The drawing under review shows one solid part. Ordinate dimensions are in mm from its lowest x, y, z. Round coordinates to 2 decimals unless told otherwise and drop trailing zeros. Order: outer loops, then holes, each group sorted by start corner. A loop starts at its lowest first (then second) coordinate and runs counter-clockwise, first axis right, second up. Notation, with made-up numbers: M 3,80 L 17,80 A24 ccw 17,114 Z; hole C 61,1.5 d8. An arc over 180 degrees is marked long. Answer in a Markdown table with one row per item. Add a question column.
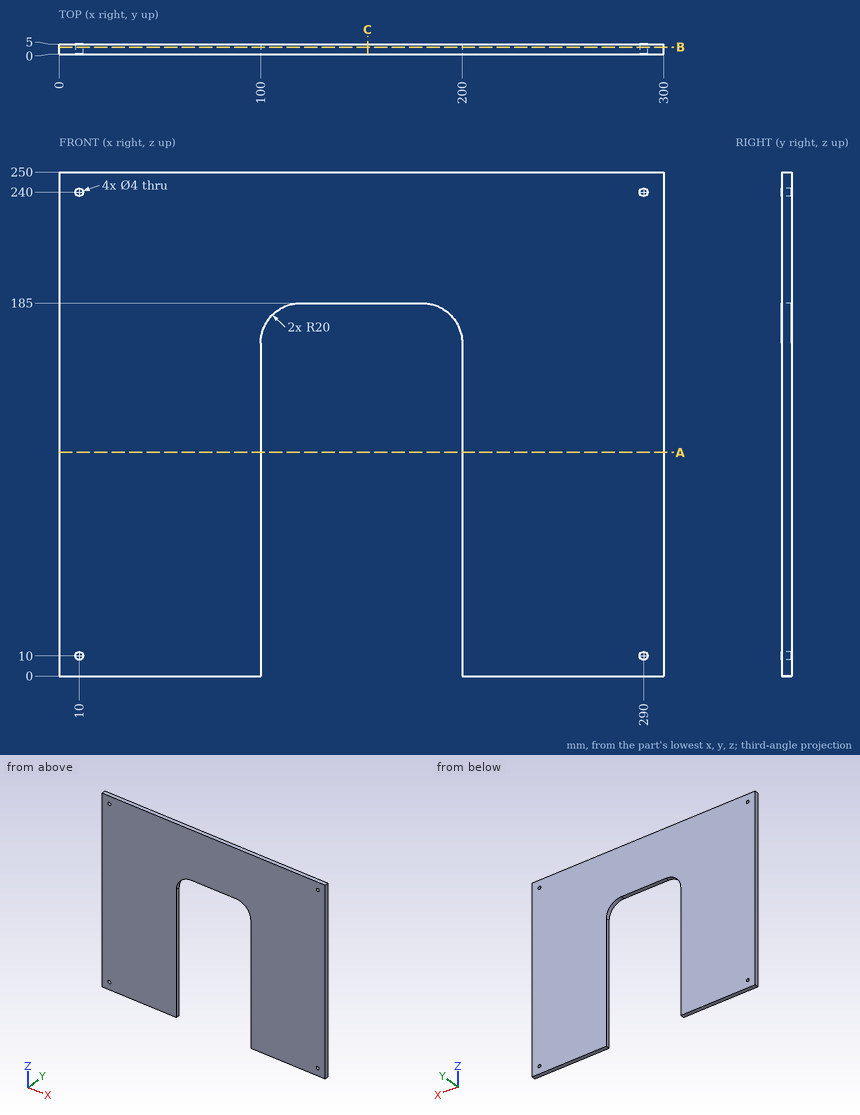
1. To check wall thickness, follow probe 1 along Z at (x, y) = (290, 2.8); probe 2 along X at (y, z) = (2.8, 10); probe 3 along X at (y, z) = (1.15, 240). State the ranges of each line that lie inside material, in increasing order. Write a range as [from, to].
2. Consider section C-C on x = 153. Write out the cut boundary in (y, z).
3. Consider section B-B on y = 3.4. Write out the cut boundary in (x, z), plus the area to 3 significant figures.
4. Clearance check with flat-ended pins moving along their axes: pin 1 Ø2.5 at (x, z) = (10, 240) entering from -Y; pin 2 Ø1.5 at (x, y) = (178.5, 1) entering from -Z. State where each tip first meets the part, or that it passes through.
5. Consider section A-A on z = 111. Write out the cut boundary in (x, y), plus the area to 3 significant figures.
Solved:
| question | item | result |
|---|---|---|
| 1 | probe 1 | z = [0, 8], [12, 238], [242, 250] |
| 1 | probe 2 | x = [0, 8], [12, 100], [200, 288], [292, 300] |
| 1 | probe 3 | x = [0, 8], [12, 288], [292, 300] |
| 2 | outline | M 0,185 L 5,185 L 5,250 L 0,250 Z |
| 3 | outline | M 0,0 L 100,0 L 100,165 A20 cw 120,185 L 180,185 A20 cw 200,165 L 200,0 L 300,0 L 300,250 L 0,250 Z; hole C 10,10 d4; hole C 10,240 d4; hole C 290,10 d4; hole C 290,240 d4 |
| 3 | area | 56,600 mm^2 |
| 4 | pin 1 | passes through |
| 4 | pin 2 | stops at z = 185 |
| 5 | outline | M 0,0 L 100,0 L 100,5 L 0,5 Z; M 200,0 L 300,0 L 300,5 L 200,5 Z |
| 5 | area | 1,000 mm^2 |
